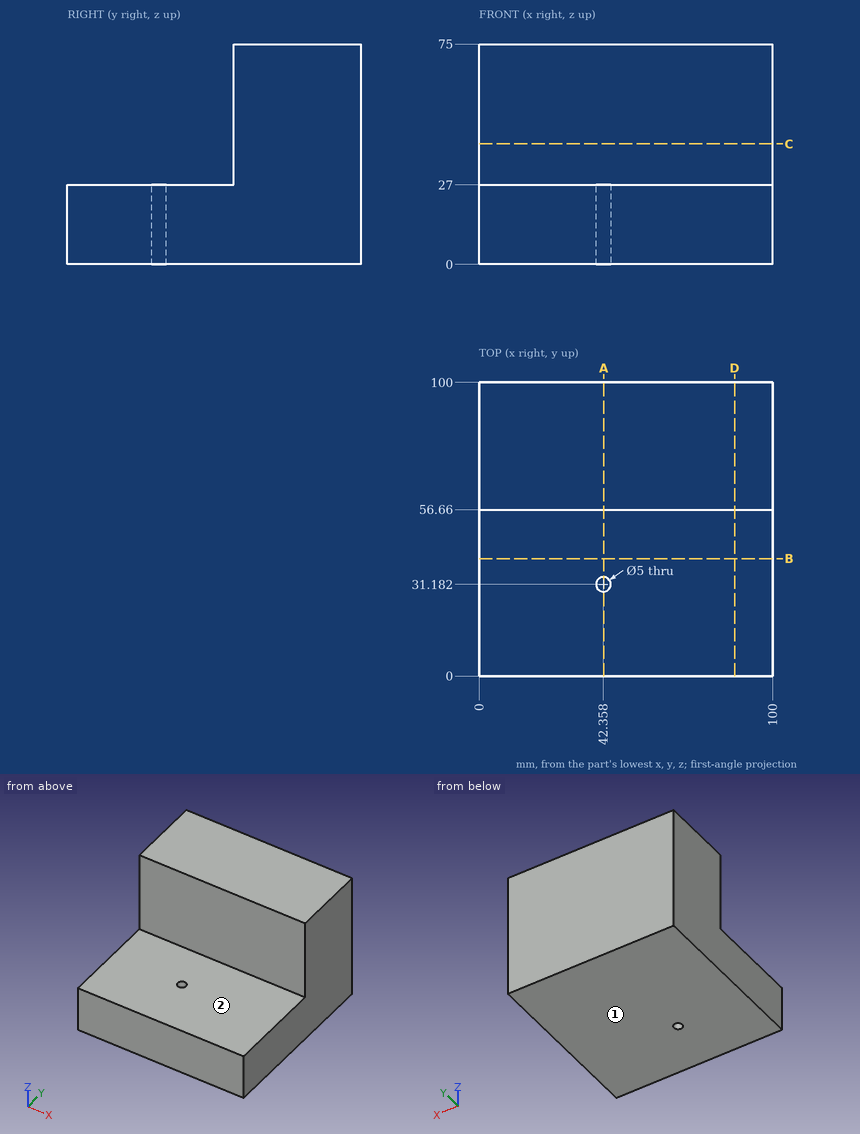
Geometry check sheet. Reference: drawing and pictorial views, mm from the part's lowest x, y, z. A direction names the side the tool comes from. Coordinates: 2 decimals unless noted, no trailing zeros. Loops run counter-clockwise (first coordinate to the right, second up) from the corner with the lowest first, then second, coordinate; pieces in that order, holes last.
1) Material ranges on probe 1 along Y at (x, z) = (56, 35); probe 2 along Z at (x, y) = (87.5, 17), recorded low to high.
2) Access from +Z, -Z, +X, -X, +Y, -Y to the whole of each face (thin tool, end or side, straight path). Record for the marked faces 1 and 2.
3) Sectioned sample at A-A (x = 42.5). Record the boundary of the cut face in (y, z), and give its area (3 significant figures).
4) Sectioned sample at C-C (z = 41). Record the boundary of the cut face in (x, y).
5) Gauge pin test, flat ends, axial feed: pin 1 (6 mm diameter, centred on x = 14.5, z = 57.5, fed in from -Y); pin 2 (17 mm diameter, centred on x = 42, y = 38, fed in from +Z). Record the tip position at first contact, or that the pin passes through.
6) Sectioned sample at D-D (x = 87). Record the boundary of the cut face in (y, z).
7) Sectioned sample at B-B (y = 40). Record the boundary of the cut face in (x, z).
Check sheet entries:
1. probe 1: y = 56.66 to 100
1. probe 2: z = 0 to 27
2. face 1: -Z, +X, -X, +Y, -Y
2. face 2: +Z, +X, -X, -Y
3. outline: (0, 0) - (28.69, 0) - (28.69, 27) - (0, 27) - close; (33.68, 0) - (100, 0) - (100, 75) - (56.66, 75) - (56.66, 27) - (33.68, 27) - close
3. area: 4,650 mm2
4. outline: (0, 56.66) - (100, 56.66) - (100, 100) - (0, 100) - close
5. pin 1: stops at y = 56.66
5. pin 2: stops at z = 27
6. outline: (0, 0) - (100, 0) - (100, 75) - (56.66, 75) - (56.66, 27) - (0, 27) - close
7. outline: (0, 0) - (100, 0) - (100, 27) - (0, 27) - close
